from build123d import *

# Parameters (mm, degrees)
EXTRUDE_THIN1_DEPTH = 31.75
SKETCH2_R           = 4.7625
CUT_EXTRUDE1_DEPTH  = 51.823787507
SKETCH3_R           = 3.175
CUT_EXTRUDE2_DEPTH  = 51.823787507
FILLET1_R           = 9.525


with BuildPart() as part:
    # Sketch1 → Extrude-Thin1 (new, symmetric)
    with BuildSketch(Plane(origin=(0, 0, 0), x_dir=(0, 0, -1), z_dir=(1, 0, 0))):
        Polygon((-8.895267484, 23.791473607), (0, 0), (0, -38.1), (-2.3622, -38.1), (-2.3622, -0.427155344), (-11.107874529, 22.964213731), align=None)
    extrude(amount=EXTRUDE_THIN1_DEPTH, both=True)

    # Sketch2 → Cut-Extrude1 (cut, through all)
    with BuildSketch(Plane(origin=(0, 0, 0), x_dir=(-1, 0, 0), z_dir=(0, 0, -1))):
        with Locations(Location((12.7, -22.225, 0), (0, 0, 90))):
            Circle(SKETCH2_R)
    extrude(amount=-CUT_EXTRUDE1_DEPTH, mode=Mode.SUBTRACT)

    # Sketch3 → Cut-Extrude2 (cut, through all)
    with BuildSketch(Plane(origin=(0, 0, 0), x_dir=(-1, 0, 0), z_dir=(0, 0.35020738125946876, -0.9366721892483971))):
        with Locations(Location((-22.225, 15.875, 0), (0, 0, 90))):
            Circle(SKETCH3_R)
        with Locations(Location((22.225, 15.875, 0), (0, 0, 90))):
            Circle(SKETCH3_R)
    extrude(amount=-CUT_EXTRUDE2_DEPTH, mode=Mode.SUBTRACT)

    # Fillet1
    fillet1_edges = [part.edges().sort_by_distance(p)[0] for p in [
        (31.75, 23.377843669, 10.001571007),
        (-31.75, 23.377843669, 10.001571007),
        (-31.75, -38.1, 1.1811),
        (31.75, -38.1, 1.1811),
    ]]
    fillet(fillet1_edges, radius=FILLET1_R)


solid = part.part
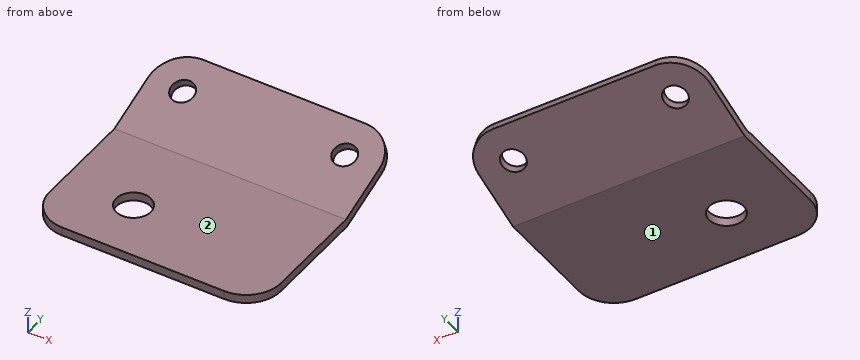
Geometry check sheet. Reference: the model listing, model coordinates, mm. Face numbers are marked on the shaded views. A direction names the side the tool comes from. Round coordinates to 2 decimals unless told otherwise and drop trailing zeros. Write each loop counter-clockwise with the first axis right and the second up, starting at its lowest first coordinate (ties: lowest second). Pieces come first, ordered by that corner, then holes.
Item 1: Section check A-A (x = -12.7). Record the boundary of the cut face in (y, z), plus the area to 3 significant figures.
Determined:
outline: (-38.1, 0) - (-26.99, 0) - (-26.99, 2.36) - (-38.1, 2.36) - close; (-17.46, 0) - (0, 0) - (23.79, 8.9) - (22.96, 11.11) - (-0.43, 2.36) - (-17.46, 2.36) - close
area: 126 mm2
Item 2: Section check B-B (y = -19). Record the boundary of the cut face in (x, z), plus the area to 3 significant figures.
Determined:
outline: (-31.75, 0) - (-16.2, 0) - (-16.2, 2.36) - (-31.75, 2.36) - close; (-9.2, 0) - (31.75, 0) - (31.75, 2.36) - (-9.2, 2.36) - close
area: 133 mm2
Item 3: Material ranges on line 1 along X through (y, z) = (13, 6.75); line 2 along Z through (x, y) = (17, -7.5); line 3 along Z through (x, y) = (28.5, 6), recorded low to high.
Determined:
line 1: x = -31.75 to -25.11, -19.34 to 19.34, 25.11 to 31.75
line 2: z = 0 to 2.36
line 3: z = 2.24 to 4.77
Item 4: Access from +Z, -Z, +X, -X, +Y, -Y to the whole of each face (thin tool, end or side, straight path). Record for the marked faces 1 and 2.
Determined:
face 1: -Z, +X, -X, +Y, -Y
face 2: +Z, +X, -X, -Y
Item 5: Section check C-C (x = 9.5). Record the boundary of the cut face in (y, z).
Determined:
outline: (-38.1, 0) - (0, 0) - (23.79, 8.9) - (22.96, 11.11) - (-0.43, 2.36) - (-38.1, 2.36) - close
Item 6: Go/stop test with flat-tipped pins: pin 1 Ø5 at (x, y) = (2, 5.5) entering from -Z; pin 2 Ø4 at (x, y) = (21.5, 8) entering from -Z; pin 3 Ø1 at (x, y) = (16, 1.5) entering from +Z. Record where each tip stops, or that it passes through.
Determined:
pin 1: stops at z = 1.12
pin 2: stops at z = 2.24
pin 3: stops at z = 3.27
